from build123d import *

# Parameters (mm, degrees)
BOSS_EXTRUDE1_DEPTH           = 2
BOSS_EXTRUDE2_DEPTH           = 8.5
CUT_EXTRUDE1_DEPTH            = 1.5
BOSS_EXTRUDE3_DEPTH           = 6.5
BOSS_EXTRUDE4_START           = 6.5
BOSS_EXTRUDE4_DEPTH           = 3
BOSS_EXTRUDE4_DRAFT           = 10
BOSS_EXTRUDE4_PROFILE_2_DEPTH = 3
BOSS_EXTRUDE4_PROFILE_2_DRAFT = 10
BOSS_EXTRUDE4_PROFILE_3_DEPTH = 3
BOSS_EXTRUDE4_PROFILE_3_DRAFT = 10
FILLET1_R                     = 3
FILLET2_R                     = 2


with BuildPart() as part:
    # Sketch1 → Boss-Extrude1 (new body)
    with BuildSketch(Plane(origin=(0, 0, 0), x_dir=(1, 0, 0), z_dir=(0, 1, 0))):
        with BuildLine():
            Line((-54.401224723, -30.978253121), (30.098775277, -30.978253121))
            ThreePointArc((30.098775277, -30.978253121), (32.220095621, -30.099573464), (33.098775277, -27.978253121))
            Line((33.098775277, -27.978253121), (33.098775277, 26.967561283))
            ThreePointArc((33.098775277, 26.967561283), (32.220095621, 29.088881626), (30.098775277, 29.967561283))
            Line((30.098775277, 29.967561283), (-54.401224723, 29.967561283))
            ThreePointArc((-54.401224723, 29.967561283), (-56.522545066, 29.088881626), (-57.401224723, 26.967561283))
            Line((-57.401224723, 26.967561283), (-57.401224723, -27.978253121))
            ThreePointArc((-57.401224723, -27.978253121), (-56.522545066, -30.099573464), (-54.401224723, -30.978253121))
        make_face()
    extrude(amount=BOSS_EXTRUDE1_DEPTH)

    # Sketch1<3> → Boss-Extrude2 (add)
    with BuildSketch(Plane(origin=(0, 0, 0), x_dir=(1, 0, 0), z_dir=(0, 1, 0))):
        with BuildLine():
            Line((-54.401224723, 31.967561283), (30.098775277, 31.967561283))
            ThreePointArc((30.098775277, 31.967561283), (33.634309183, 30.503095189), (35.098775277, 26.967561283))
            Line((35.098775277, 26.967561283), (35.098775277, -27.978253121))
            ThreePointArc((35.098775277, -27.978253121), (33.634309183, -31.513787026), (30.098775277, -32.978253121))
            Line((30.098775277, -32.978253121), (-54.401224723, -32.978253121))
            ThreePointArc((-54.401224723, -32.978253121), (-57.936758629, -31.513787026), (-59.401224723, -27.978253121))
            Line((-59.401224723, -27.978253121), (-59.401224723, 26.967561283))
            ThreePointArc((-59.401224723, 26.967561283), (-57.936758629, 30.503095189), (-54.401224723, 31.967561283))
        make_face()
        with BuildLine():
            Line((-54.401224723, -30.978253121), (30.098775277, -30.978253121))
            ThreePointArc((30.098775277, -30.978253121), (32.220095621, -30.099573464), (33.098775277, -27.978253121))
            Line((33.098775277, -27.978253121), (33.098775277, 26.967561283))
            ThreePointArc((33.098775277, 26.967561283), (32.220095621, 29.088881626), (30.098775277, 29.967561283))
            Line((30.098775277, 29.967561283), (-54.401224723, 29.967561283))
            ThreePointArc((-54.401224723, 29.967561283), (-56.522545066, 29.088881626), (-57.401224723, 26.967561283))
            Line((-57.401224723, 26.967561283), (-57.401224723, -27.978253121))
            ThreePointArc((-57.401224723, -27.978253121), (-56.522545066, -30.099573464), (-54.401224723, -30.978253121))
        make_face(mode=Mode.SUBTRACT)
    extrude(amount=BOSS_EXTRUDE2_DEPTH)

    # Sketch2 → Cut-Extrude1 (cut)
    with BuildSketch(Plane(origin=(0, 8.5, 0), x_dir=(1, 0, 0), z_dir=(0, 1, 0))):
        with BuildLine():
            Line((27.798775277, -25.532438717), (27.798775277, 27.567561283))
            ThreePointArc((27.798775277, 27.567561283), (26.861516977, 29.830302983), (24.598775277, 30.767561283))
            Line((24.598775277, 30.767561283), (-54.401224723, 30.767561283))
            ThreePointArc((-54.401224723, 30.767561283), (-56.663966423, 29.830302983), (-57.601224723, 27.567561283))
            Line((-57.601224723, 27.567561283), (-57.601224723, -22.332438717))
            ThreePointArc((-57.601224723, -22.332438717), (-56.663966423, -24.595180417), (-54.401224723, -25.532438717))
            Line((-54.401224723, -25.532438717), (27.798775277, -25.532438717))
        make_face()
    extrude(amount=-CUT_EXTRUDE1_DEPTH, mode=Mode.SUBTRACT)

    # Sketch3 → Boss-Extrude3 (add)
    with BuildSketch(Plane(origin=(0, 2, 0), x_dir=(1, 0, 0), z_dir=(0, 1, 0))):
        with BuildLine():
            Line((28.932049088, -29.286400666), (31.406922822, -26.811526932))
            Line((31.406922822, -26.811526932), (33.198775277, -26.811526932))
            Line((33.198775277, -26.811526932), (33.198775277, -27.978253121))
            ThreePointArc((33.198775277, -27.978253121), (32.290806299, -30.170284142), (30.098775277, -31.078253121))
            Line((30.098775277, -31.078253121), (28.932049088, -31.078253121))
            Line((28.932049088, -31.078253121), (28.932049088, -29.286400666))
        make_face()
        with BuildLine():
            Line((31.406922822, 25.800835094), (28.932049088, 28.275708828))
            Line((28.932049088, 28.275708828), (28.932049088, 30.067561283))
            Line((28.932049088, 30.067561283), (30.098775277, 30.067561283))
            ThreePointArc((30.098775277, 30.067561283), (32.290806299, 29.159592304), (33.198775277, 26.967561283))
            Line((33.198775277, 26.967561283), (33.198775277, 25.800835094))
            Line((33.198775277, 25.800835094), (31.406922822, 25.800835094))
        make_face()
        with BuildLine():
            Line((-53.234498534, -29.286400666), (-55.709372268, -26.811526932))
            Line((-55.709372268, -26.811526932), (-57.501224723, -26.811526932))
            Line((-57.501224723, -26.811526932), (-57.501224723, -27.978253121))
            ThreePointArc((-57.501224723, -27.978253121), (-56.593255745, -30.170284142), (-54.401224723, -31.078253121))
            Line((-54.401224723, -31.078253121), (-53.234498534, -31.078253121))
            Line((-53.234498534, -31.078253121), (-53.234498534, -29.286400666))
        make_face()
    extrude(amount=BOSS_EXTRUDE3_DEPTH)


with BuildPart() as boss_extrude4_tool:
    # Sketch3<2> → Boss-Extrude4 (with draft: the straight prism first)
    with BuildSketch(Plane(origin=(0, 2, 0), x_dir=(1, 0, 0), z_dir=(0, 1, 0)).offset(BOSS_EXTRUDE4_START)):
        with BuildLine():
            Line((28.932049088, -29.286400666), (28.932049088, -31.078253121))
            Line((28.932049088, -31.078253121), (30.098775277, -31.078253121))
            ThreePointArc((30.098775277, -31.078253121), (32.290806299, -30.170284142), (33.198775277, -27.978253121))
            Line((33.198775277, -27.978253121), (33.198775277, -26.811526932))
            Line((33.198775277, -26.811526932), (31.406922822, -26.811526932))
            Line((31.406922822, -26.811526932), (28.932049088, -29.286400666))
        make_face()
    extrude(amount=BOSS_EXTRUDE4_DEPTH)
    # Boss-Extrude4: the draft: its side faces are tilted about the plane it starts from
    boss_extrude4_sides = [boss_extrude4_tool.faces().sort_by_distance(p)[0] for p in [
        (28.932049088, 10, 30.182326893),
        (29.515412183, 10, 31.078253121),
        (32.290806299, 10, 30.170284142),
        (33.198775277, 10, 27.394890026),
        (32.30284905, 10, 26.811526932),
        (30.169485955, 10, 28.048963799),
    ]]
    draft(boss_extrude4_sides, Plane(origin=(0, 2, 0), x_dir=(1, 0, 0), z_dir=(0, 1, 0)).offset(BOSS_EXTRUDE4_START), BOSS_EXTRUDE4_DRAFT)


with BuildPart() as part_1:
    add(part.part)

    # Boss-Extrude4: add boss_extrude4_tool
    add(boss_extrude4_tool.part)


with BuildPart() as boss_extrude4_profile_2_tool:
    # Sketch3<2> → Boss-Extrude4 profile 2 (with draft: the straight prism first)
    with BuildSketch(Plane(origin=(0, 2, 0), x_dir=(1, 0, 0), z_dir=(0, 1, 0)).offset(BOSS_EXTRUDE4_START)):
        with BuildLine():
            Line((31.406922822, 25.800835094), (33.198775277, 25.800835094))
            Line((33.198775277, 25.800835094), (33.198775277, 26.967561283))
            ThreePointArc((33.198775277, 26.967561283), (32.290806299, 29.159592304), (30.098775277, 30.067561283))
            Line((30.098775277, 30.067561283), (28.932049088, 30.067561283))
            Line((28.932049088, 30.067561283), (28.932049088, 28.275708828))
            Line((28.932049088, 28.275708828), (31.406922822, 25.800835094))
        make_face()
    extrude(amount=BOSS_EXTRUDE4_PROFILE_2_DEPTH)
    # Boss-Extrude4 profile 2: the draft: its side faces are tilted about the plane it starts from
    boss_extrude4_profile_2_sides = [boss_extrude4_profile_2_tool.faces().sort_by_distance(p)[0] for p in [
        (32.30284905, 10, -25.800835094),
        (33.198775277, 10, -26.384198188),
        (32.290806299, 10, -29.159592304),
        (29.515412183, 10, -30.067561283),
        (28.932049088, 10, -29.171635055),
        (30.169485955, 10, -27.038271961),
    ]]
    draft(boss_extrude4_profile_2_sides, Plane(origin=(0, 2, 0), x_dir=(1, 0, 0), z_dir=(0, 1, 0)).offset(BOSS_EXTRUDE4_START), BOSS_EXTRUDE4_PROFILE_2_DRAFT)


with BuildPart() as part_2:
    add(part_1.part)

    # Boss-Extrude4 profile 2: add boss_extrude4_profile_2_tool
    add(boss_extrude4_profile_2_tool.part)


with BuildPart() as boss_extrude4_profile_3_tool:
    # Sketch3<2> → Boss-Extrude4 profile 3 (with draft: the straight prism first)
    with BuildSketch(Plane(origin=(0, 2, 0), x_dir=(1, 0, 0), z_dir=(0, 1, 0)).offset(BOSS_EXTRUDE4_START)):
        with BuildLine():
            Line((-53.234498534, -29.286400666), (-55.709372268, -26.811526932))
            Line((-55.709372268, -26.811526932), (-57.501224723, -26.811526932))
            Line((-57.501224723, -26.811526932), (-57.501224723, -27.978253121))
            ThreePointArc((-57.501224723, -27.978253121), (-56.593255745, -30.170284142), (-54.401224723, -31.078253121))
            Line((-54.401224723, -31.078253121), (-53.234498534, -31.078253121))
            Line((-53.234498534, -31.078253121), (-53.234498534, -29.286400666))
        make_face()
    extrude(amount=BOSS_EXTRUDE4_PROFILE_3_DEPTH)
    # Boss-Extrude4 profile 3: the draft: its side faces are tilted about the plane it starts from
    boss_extrude4_profile_3_sides = [boss_extrude4_profile_3_tool.faces().sort_by_distance(p)[0] for p in [
        (-54.471935401, 10, 28.048963799),
        (-56.605298496, 10, 26.811526932),
        (-57.501224723, 10, 27.394890026),
        (-56.593255745, 10, 30.170284142),
        (-53.817861628, 10, 31.078253121),
        (-53.234498534, 10, 30.182326893),
    ]]
    draft(boss_extrude4_profile_3_sides, Plane(origin=(0, 2, 0), x_dir=(1, 0, 0), z_dir=(0, 1, 0)).offset(BOSS_EXTRUDE4_START), BOSS_EXTRUDE4_PROFILE_3_DRAFT)


with BuildPart() as part_3:
    add(part_2.part)

    # Boss-Extrude4 profile 3: add boss_extrude4_profile_3_tool
    add(boss_extrude4_profile_3_tool.part)

    # Fillet1
    fillet1_edges = [part_3.edges().sort_by_distance(p)[0] for p in [
        (-12.151224723, 0, -31.967561283),
        (33.634309183, 0, -30.503095189),
        (35.098775277, 0, 0.505345919),
        (33.634309183, 0, 31.513787026),
        (-12.151224723, 0, 32.978253121),
        (-57.936758629, 0, 31.513787026),
        (-59.401224723, 0, 0.505345919),
        (-57.936758629, 0, -30.503095189),
    ]]
    fillet(fillet1_edges, radius=FILLET1_R)

    # Fillet2
    fillet2_edges = [part_3.edges().sort_by_distance(p)[0] for p in [
        (-56.522545066, 2, -29.088881626),
        (33.098775277, 2, 0.505345919),
        (32.25284905, 2, 26.811526932),
        (30.169485955, 2, 28.048963799),
        (28.932049088, 2, 30.132326893),
        (-57.401224723, 2, -0.078017176),
        (-12.151224723, 2, 30.978253121),
        (-53.234498534, 2, 30.132326893),
        (-54.471935401, 2, 28.048963799),
        (-12.734587817, 2, -29.967561283),
        (-56.555298496, 2, 26.811526932),
        (28.932049088, 2, -29.121635055),
        (30.169485955, 2, -27.038271961),
        (32.25284905, 2, -25.800835094),
    ]]
    fillet(fillet2_edges, radius=FILLET2_R)


solid = part_3.part
Can you work these out from the model? Positions are in its coordinate system, mm. A direction names the side the tool comes from. Coordinates: 2 decimals unless noted, no trailing zeros. Write each loop counter-clockwise with the first axis right and the second up, starting at its lowest first coordinate (ties: lowest second). Pieces come first, ordered by that corner, then holes.
Q1. Please list where these lines run through material, in increasing order: L1, parallel to Z at x = -23.5, y = 6.5; L2, parallel to X at y = 8, z = 17; L3, parallel to X at y = 5.25, z = -18.
Results found:
L1: z = -31.97 to -29.97, 30.98 to 32.98
L2: x = -59.4 to -57.6, 33.1 to 35.1
L3: x = -59.4 to -57.4, 33.1 to 35.1
Q2. For P1, Ø1.9, axis at y = 7.5, z = 30.5, coming from the +X side; P2, Ø1.9, axis at x = 32, y = 5, coming from the +Z side; P3, Ø1.9, axis at x = 32.5, y = 6.5, coming from the -Z side, each with a flat end and sliding along its axis, tell me the tip position at first contact or that it passes through.
Results found:
P1: stops at x = 34.85
P2: stops at z = 32.89
P3: stops at z = -31.75
Q3. Imagine slicing it at B-B, the plane z = -14. List the corners of the cut face in (x, y) for me, plus the area to 3 significant figures.
Results found:
outline: (-59.4, 3) arc R3 ccw to (-56.4, 0) - (32.1, 0) arc R3 ccw to (35.1, 3) - (35.1, 8.5) - (33.1, 8.5) - (33.1, 4) arc R2 cw to (31.1, 2) - (-55.4, 2) arc R2 cw to (-57.4, 4) - (-57.4, 7) - (-57.6, 7) - (-57.6, 8.5) - (-59.4, 8.5) - close
area: 213 mm2
Q4. If we mould it in two halves opening along X, with no side actions, what happens to faces 1 (the face through (33.595, 5.712, -30.542)), 2 (the face through (-56.431, 9.979, 29.964)), 3 (the face through (28.558, 2.835, -28.725))? For each: +X half, -X half, draft (parallel to the pull), parting line (faces both ways), or undercut.
Results found:
face 1: +X half
face 2: -X half
face 3: undercut
Q5. Which directions (+Z, -Z, +X, -X, +Y, -Y) give clear straight access to the entire face, cutting with the end or side of a thin tool? Please do faces 4 (the face through (-55, 11.5, 29)), 5 (the face through (-54.64, 9.98, 28.25)), 6 (the face through (31.856, 2.835, 26.437)).
Results found:
face 4: +Z, -Z, +X, -X, +Y
face 5: -Z, +Y
face 6: +Y
Q6. Imagine slicing it at C-C, the plane x = -28. List the corners of the cut face in (y, z) for me, plus the area to 3 significant figures.
Results found:
outline: (0, -28.97) arc R3 ccw to (3, -31.97) - (8.5, -31.97) - (8.5, -30.77) - (7, -30.77) - (7, -29.97) - (4, -29.97) arc R2 cw to (2, -27.97) - (2, 28.98) arc R2 cw to (4, 30.98) - (8.5, 30.98) - (8.5, 32.98) - (3, 32.98) arc R3 ccw to (0, 29.98) - close
area: 153 mm2
Q7. Imagine slicing it at A-A, the plane y = 5.25. List the corners of the cut face in (x, z) for me.
Results found:
outline: (-59.4, -26.97) arc R5 ccw to (-54.4, -31.97) - (30.1, -31.97) arc R5 ccw to (35.1, -26.97) - (35.1, 27.98) arc R5 ccw to (30.1, 32.98) - (-54.4, 32.98) arc R5 ccw to (-59.4, 27.98) - close; hole (-57.4, -26.97) arc R3 ccw to (-54.4, -29.97) - (28.93, -29.97) - (28.93, -28.28) - (31.41, -25.8) - (33.1, -25.8) - (33.1, 26.81) - (31.41, 26.81) - (28.93, 29.29) - (28.93, 30.98) - (-53.23, 30.98) - (-53.23, 29.29) - (-55.71, 26.81) - (-57.4, 26.81) - close
